```python
from build123d import *

# Parameters (mm, degrees)
BOSS_EXTRUDE1_DEPTH     = 3
BOSS_EXTRUDE2_DEPTH     = 6
SKETCH3_R               = 1.6
BOSS_EXTRUDE3_DEPTH     = 3
MIRROR2_COPY_1_DEPTH    = 6
MIRROR2_COPY_2_SKETCH_R = 1.6
MIRROR2_COPY_2_DEPTH    = 3


with BuildPart() as part:
    # Sketch1 → Boss-Extrude1 (new body)
    with BuildSketch(Plane.XY):
        with BuildLine():
            Line((-71.122052126, 155), (-71.122052126, 71))
            ThreePointArc((-71.122052126, 71), (-69.071799594, 66.050252532), (-64.122052126, 64))
            Line((-64.122052126, 64), (39.877947874, 64))
            ThreePointArc((39.877947874, 64), (44.827695342, 66.050252532), (46.877947874, 71))
            Line((46.877947874, 71), (46.877947874, 155))
            ThreePointArc((46.877947874, 155), (44.827695342, 159.949747468), (39.877947874, 162))
            Line((39.877947874, 162), (-64.122052126, 162))
            ThreePointArc((-64.122052126, 162), (-69.071799594, 159.949747468), (-71.122052126, 155))
        make_face()
    extrude(amount=-BOSS_EXTRUDE1_DEPTH)

    # Sketch2 → Boss-Extrude2 (add)
    with BuildSketch(Plane(origin=(0, 0, -3), x_dir=(-1, 0, 0), z_dir=(0, 0, -1))):
        with BuildLine():
            Line((-46.768394201, 156.233592078), (-43.877947874, 153.343145751))
            Line((-43.877947874, 153.343145751), (-43.877947874, 155))
            ThreePointArc((-43.877947874, 155), (-42.706374999, 157.828427125), (-39.877947874, 159))
            Line((-39.877947874, 159), (-38.221093625, 159))
            Line((-38.221093625, 159), (-41.111539952, 161.890446327))
            ThreePointArc((-41.111539952, 161.890446327), (-44.827695342, 159.949747468), (-46.768394201, 156.233592078))
        make_face()
    boss_extrude2 = extrude(amount=BOSS_EXTRUDE2_DEPTH)

    # Sketch3 → Boss-Extrude3 (add)
    with BuildSketch(Plane(origin=(0, 0, -9), x_dir=(-1, 0, 0), z_dir=(0, 0, -1))):
        with BuildLine():
            Line((-43.877947874, 153.343145751), (-43.877947874, 155))
            ThreePointArc((-43.877947874, 155), (-42.706374999, 157.828427125), (-39.877947874, 159))
            Line((-39.877947874, 159), (-38.221093625, 159))
            Line((-38.221093625, 159), (-47.656122467, 168.435028843))
            ThreePointArc((-47.656122467, 168.435028843), (-53.312976717, 168.435028843), (-53.312976717, 162.778174593))
            Line((-53.312976717, 162.778174593), (-43.877947874, 153.343145751))
        make_face()
        with Locations((-50.484549592, 165.606601718)):
            Circle(SKETCH3_R, mode=Mode.SUBTRACT)
    boss_extrude3 = extrude(amount=BOSS_EXTRUDE3_DEPTH)

    # Mirror1: Boss-Extrude2, Boss-Extrude3 across plane
    add(boss_extrude2.mirror(Plane.ZY.offset(12.122052126)))
    add(boss_extrude3.mirror(Plane.ZY.offset(12.122052126)))

    # Mirror2: Boss-Extrude2, Boss-Extrude3 across plane
    add(boss_extrude2.mirror(Plane.ZX.offset(113)))
    add(boss_extrude3.mirror(Plane.ZX.offset(113)))

    # Mirror2 copy 1 sketch → Mirror2 copy 1 (add)
    with BuildSketch(Plane(origin=(-24.244104252, 226, -3), x_dir=(1, 0, 0), z_dir=(0, 0, -1))):
        with BuildLine():
            Line((-46.768394201, 156.233592078), (-43.877947874, 153.343145751))
            Line((-43.877947874, 153.343145751), (-43.877947874, 155))
            ThreePointArc((-43.877947874, 155), (-42.706374999, 157.828427125), (-39.877947874, 159))
            Line((-39.877947874, 159), (-38.221093625, 159))
            Line((-38.221093625, 159), (-41.111539952, 161.890446327))
            ThreePointArc((-41.111539952, 161.890446327), (-44.827695342, 159.949747468), (-46.768394201, 156.233592078))
        make_face()
    extrude(amount=MIRROR2_COPY_1_DEPTH)

    # Mirror2 copy 2 sketch → Mirror2 copy 2 (add)
    with BuildSketch(Plane(origin=(-24.244104252, 226, -9), x_dir=(1, 0, 0), z_dir=(0, 0, -1))):
        with BuildLine():
            Line((-43.877947874, 153.343145751), (-43.877947874, 155))
            ThreePointArc((-43.877947874, 155), (-42.706374999, 157.828427125), (-39.877947874, 159))
            Line((-39.877947874, 159), (-38.221093625, 159))
            Line((-38.221093625, 159), (-47.656122467, 168.435028843))
            ThreePointArc((-47.656122467, 168.435028843), (-53.312976717, 168.435028843), (-53.312976717, 162.778174593))
            Line((-53.312976717, 162.778174593), (-43.877947874, 153.343145751))
        make_face()
        with Locations((-50.484549592, 165.606601718)):
            Circle(MIRROR2_COPY_2_SKETCH_R, mode=Mode.SUBTRACT)
    extrude(amount=MIRROR2_COPY_2_DEPTH)


solid = part.part
```
Input: part model. Units: mm. Frame: model coordinates. A direction names the side the tool comes from. Coordinates: 2 decimals unless noted, no trailing zeros. Loops run counter-clockwise (first coordinate to the right, second up) from the corner with the lowest first, then second, coordinate; pieces in that order, holes last. Notation, with made-up numbers: M 51.5,65.5 L 95.5,65.5 A29 ccw 95.5,89.5 Z; hole C 54,42 d6. An arc over 180 degrees is marked long. Use a Markdown table: item, result. Add a question column.
1) Line query: L1, parallel to Z at x = -55.5, y = 101; L2, parallel to Y at x = 12, z = -2.5; L3, parallel to X at y = 117.5, z = -2.25. Output: solid intervals per line, ascending. Write a range as from..to.
2) Section B-B, the plane x = -24.5. Return the cut outline in (y, z).
3) Section A-A, the plane z = -6.5. Return the cut outline in (x, y), plus the area to 3 significant figures.
4) Draft query along Y for faces 5 (the flat face through (-71.122, 114, -1)), 6 (the flat face through (-13, 64, -1)), 7 (the cylindrical face through (-66.98, 68.2, -7.44)). Return one class per face: +Y half, -Y half, draft (parallel to the pull), parting line (faces both ways), or undercut.
5) Section C-C, the plane y = 118. Return the cut outline in (x, z), plus the area to 3 significant figures.
6) Set-up query: faces 1 (the flat face through (49, 63, -9)), 2 (the flat face through (-74, 63, -9)), 3 (the cylindrical face through (42.737, 157.797, -7.437)), 4 (the flat face through (-74, 163, -9)). Return all of +Z, -Z, +X, -X, +Y, -Y with unobstructed straight access to the full face (end or side cutting, diameter ignored); none if empty.
7) Pin query (flat end, axial travel): P1, Ø5, axis at x = 50.48, y = 165.61, coming from the +Z side; P2, Ø1.3, axis at x = 39, z = -9, coming from the +Y side; P3, Ø4, axis at y = 97.5, z = -2.5, coming from the +X side. Return the tip coordinate at first contact, or that it passes through.
Answer below:
| question | item | result |
|---|---|---|
| 1 | L1 | -3..0 |
| 1 | L2 | 64..162 |
| 1 | L3 | -71.12..46.88 |
| 2 | outline | M 64,-3 L 162,-3 L 162,0 L 64,0 Z |
| 3 | outline | M -71.01,69.77 A7 ccw -65.36,64.11 L -62.47,67 L -64.12,67 A4 cw -68.12,71 L -68.12,72.66 Z; M -71.01,156.23 L -68.12,153.34 L -68.12,155 A4 cw -64.12,159 L -62.47,159 L -65.36,161.89 A7 ccw Z; M 38.22,67 L 41.11,64.11 A7 ccw 46.77,69.77 L 43.88,72.66 L 43.88,71 A4 cw 39.88,67 Z; M 38.22,159 L 39.88,159 A4 cw 43.88,155 L 43.88,153.34 L 46.77,156.23 A7 ccw 41.11,161.89 Z |
| 3 | area | 108 mm2 |
| 4 | face 5 | draft |
| 4 | face 6 | -Y half |
| 4 | face 7 | undercut |
| 5 | outline | M -71.12,-3 L 46.88,-3 L 46.88,0 L -71.12,0 Z |
| 5 | area | 354 mm2 |
| 6 | face 1 | +Z, +X, -Y |
| 6 | face 2 | +Z, -X, -Y |
| 6 | face 3 | -Z |
| 6 | face 4 | +Z, -X, +Y |
| 7 | P1 | z = -9 |
| 7 | P2 | y = 160.43 |
| 7 | P3 | x = 46.88 |
